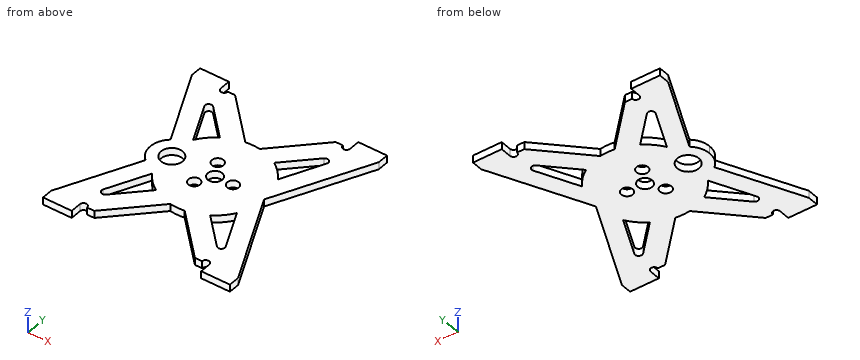
```python
from build123d import *

# Parameters (mm, degrees)
PAD_DEPTH     = 1
SKETCH008_R   = 0.8
SKETCH008_R_2 = 1
SKETCH008_R_3 = 1.5
POCKET_DEPTH  = 1.001


with BuildPart() as part:
    # Sketch007 → Pad (new body)
    with BuildSketch(Plane.XY):
        with BuildLine():
            Line((-13, 14.5), (-9, 14.5))
            Line((-9, 14.5), (-9, 13))
            ThreePointArc((-9, 13), (-8.5, 12.5), (-8, 13))
            Line((-8, 13), (-7, 13))
            Line((-7, 13), (-1, 6.928203))
            ThreePointArc((1, 6.928203), (0, 7), (-1, 6.928203))
            Line((7, 13), (1, 6.928203))
            Line((8, 13), (7, 13))
            ThreePointArc((8, 13), (8.5, 12.5), (9, 13))
            Line((9, 14.5), (9, 13))
            Line((9, 14.5), (13, 14.5))
            Line((13, 14.5), (13, 13))
            Line((6.83213, 0), (13, 13))
            Line((6.83213, 0), (-6.83213, 0))
            Line((-9, 0), (-6.83213, 0))
            ThreePointArc((-7.924155, 2.301657), (-8.717762, 1.270341), (-9, 0))
            Line((-7.924155, 2.301657), (-13, 13))
            Line((-13, 14.5), (-13, 13))
        make_face()
        with BuildLine():
            Line((-8.526013, 9.328003), (-5.892862, 3.778118))
            ThreePointArc((-3.770099, 5.897996), (-4.94638, 4.953113), (-5.892862, 3.778118))
            Line((-7.718628, 9.893773), (-3.770099, 5.897996))
            ThreePointArc((-7.718628, 9.893773), (-8.361214, 9.951801), (-8.526013, 9.328003))
        make_face(mode=Mode.SUBTRACT)
        with BuildLine():
            ThreePointArc((5.892862, 3.778118), (4.94638, 4.953113), (3.770099, 5.897996))
            Line((7.718628, 9.893773), (3.770099, 5.897996))
            ThreePointArc((8.526013, 9.328002), (8.361214, 9.951801), (7.718628, 9.893773))
            Line((8.526013, 9.328002), (5.892862, 3.778118))
        make_face(mode=Mode.SUBTRACT)
    pad = extrude(amount=PAD_DEPTH)

    # Mirrored: Pad across Sketch007 H_Axis
    add(pad.mirror(Plane.ZX))

    # Sketch008 → Pocket (cut, through all)
    with BuildSketch(Plane.XY):
        with Locations((2.5, 0)):
            Circle(SKETCH008_R)
        with Locations((-1.25, -2.165064)):
            Circle(SKETCH008_R)
        with Locations((-1.25, 2.165064)):
            Circle(SKETCH008_R)
        Circle(SKETCH008_R_2)
        with Locations((-6, 0)):
            Circle(SKETCH008_R_3)
    extrude(amount=POCKET_DEPTH, mode=Mode.SUBTRACT)


solid = part.part
```
Can you work these out from the model? Positions are in its coordinate system, mm. Coordinates: 2 decimals unless noted, no trailing zeros. Loops run counter-clockwise (first coordinate to the right, second up) from the corner with the lowest first, then second, coordinate; pieces in that order, holes last. Notation, with made-up numbers: (13, 65.5) -> (45, 65.5) arc R14 cw to (45, 84.5) -> close; hole circle Ø4 at (-7, -26). An arc over 180 degrees is marked (long way). Put each result on its own line as item: value. Start each with the question number.
Q1. I want a section at C-C (x = -5). Write out the boundary of the cut face in (y, z).
Q2. I want a section at B-B (y = -4.5). Write out the boundary of the cut face in (x, z).
Q3. If I drill on line 1 (X direction, y = 0, z = 0.4); line 2 (X direction, y = 5.5, z = 0.8); line 3 (Y direction, x = -8.25, z = 0.5), over which ranges is the centre line in solid material (lowest first)? Write a range as [from, to].
Q4. I want a section at A-A (x = 0). Write out the boundary of the cut face in (y, z).
Q5. I want a section at D-D (x = -10.5). Write out the boundary of the cut face in (y, z), plus the area to 3 significant figures.
Taken from the geometry:
1. outline: (-10.98, 0) -> (-7.14, 0) -> (-7.14, 1) -> (-10.98, 1) -> close; (-4.9, 0) -> (-1.12, 0) -> (-1.12, 1) -> (-4.9, 1) -> close; (1.12, 0) -> (4.9, 0) -> (4.9, 1) -> (1.12, 1) -> close; (7.14, 0) -> (10.98, 0) -> (10.98, 1) -> (7.14, 1) -> close
2. outline: (-8.97, 0) -> (-6.24, 0) -> (-6.24, 1) -> (-8.97, 1) -> close; (-5.36, 0) -> (5.36, 0) -> (5.36, 1) -> (-5.36, 1) -> close; (6.24, 0) -> (8.97, 0) -> (8.97, 1) -> (6.24, 1) -> close
3. line 1: x = [-9, -7.5], [-4.5, -1], [1, 1.7], [3.3, 6.83]
3. line 2: x = [-9.44, -6.71], [-4.33, 4.33], [6.71, 9.44]
3. line 3: y = [-12.57, -10.01], [-8.75, -2.99], [-1.98, 1.98], [2.99, 8.75], [10.01, 12.57]
4. outline: (-7, 0) -> (-1, 0) -> (-1, 1) -> (-7, 1) -> close; (1, 0) -> (7, 0) -> (7, 1) -> (1, 1) -> close
5. outline: (-14.5, 0) -> (-7.73, 0) -> (-7.73, 1) -> (-14.5, 1) -> close; (7.73, 0) -> (14.5, 0) -> (14.5, 1) -> (7.73, 1) -> close
5. area: 13.5 mm2
